Geometry: final body of the model. Coordinates: model frame, mm. A direction names the side the tool comes from. Give positions to 0.01 mm unless a question says otherwise; leave off trailing zeros. Loops run counter-clockwise (first coordinate to the right, second up) from the corner with the lowest first, then second, coordinate; pieces in that order, holes last. Notation, with made-up numbers: (-1, 35.5) - (23, 35.5) arc R29 cw to (23, 56.5) - close; hole circle Ø2 at (-4, -21). An arc over 180 degrees is marked (long way). Use CSV: the item, a comma, the result in double quotes. Start each with the question number.
Autodesk Fusion 360 part; units mm, degrees
sketch "Sketch2" plane through (0, 0, 0) normal (0, 1, 0) x (1, 0, 0)
  line L0 (-71.8116, -9.5677) -> (91.1884, -9.5677)
  line L1 (91.1884, -9.5677) -> (91.1884, -7.5677)
  line L2 (91.1884, -7.5677) -> (-71.8116, -7.5677)
  line L3 (-71.8116, -7.5677) -> (-71.8116, -9.5677)
  line L4 (-78.3116, -11.7677) -> (97.6884, -11.7677)
  line L5 (97.6884, -11.7677) -> (97.6884, -9.5677)
  line L6 (97.6884, -9.5677) -> (-78.3116, -9.5677)
  line L7 (-78.3116, -9.5677) -> (-78.3116, -11.7677)
  dimension "d1" = 163
  dimension "d2" = 2
  dimension "d3" = 6.5
  dimension "d4" = 6.5
  dimension "d5" = 2.2
extrude "Extrude1" add sketch "Sketch2" along normal blind 145
extrude "Extrude2" cut sketch "Sketch2" along normal blind 1 contours L0 L4 L5 L6 L7
Item 1: Section B-B (z = 8.35). Output: boundary loops of the cut face in (x, y), plus the area to 3 significant figures.
Item 2: Pin query (flat end, axial travel): pin 1 Ø2.5 at (x, z) = (-1.5, 11) entering from -Y; pin 2 Ø2 at (y, z) = (61.5, 8.5) entering from +X; pin 3 Ø2 at (x, y) = (-75.5, 45.5) entering from -Z. Return the tip coordinate at first contact, or that it passes through.
Item 3: Reachability of faces 3 (the flat face through (-75, 72, 9.568)), 4 (the flat face through (11, 71, 7.568)) from +Z, -Z, +X, -X, +Y, -Y: full face, straight path, thin tool, end or side. Return the list, or none.
Item 4: Ray query, probe 1 along Y at (x, z) = (-5, 11.25); probe 2 along X at (y, z) = (114.5, 9.05). Return the intervals inside material, ascending.
Item 5: Section A-A (y = 135). Output: boundary loops of the cut face in (x, z), plus the area to 3 significant figures.
Item 6: Mould query, pull axis Y, two halves, no side actions, for faces 1 (the flat face through (94, 72, 9.568)), 2 (the flat face through (8, 145, 10)). Classes: pulls with the +Y half, pulls with the -Y half, needs draft (parallel to the pull), parting line crosses it, or undercut.
Outcome:
1,outline,"(-71.81, 0) - (91.19, 0) - (91.19, 145) - (-71.81, 145) - close"
1,area,"23,600 mm2"
2,pin 1,"stops at y = 1"
2,pin 2,"stops at x = 91.19"
2,pin 3,"stops at z = 9.57"
3,face 3,"-Z, -X, +Y, -Y"
3,face 4,"-Z, +X, -X, +Y, -Y"
4,probe 1,"y = 1 to 145"
4,probe 2,"x = -71.81 to 91.19"
5,outline,"(-78.31, 9.57) - (-71.81, 9.57) - (-71.81, 7.57) - (91.19, 7.57) - (91.19, 9.57) - (97.69, 9.57) - (97.69, 11.77) - (-78.31, 11.77) - close"
5,area,"713 mm2"
6,face 1,"needs draft"
6,face 2,"pulls with the +Y half"
